The listing builds one solid part. Answer for the finished solid, in the listing's coordinates (mm). Give positions to 0.01 mm unless a question says otherwise; leave off trailing zeros. Order: outer loops, then holes, each group sorted by start corner. A loop starts at its lowest first (then second) coordinate and runs counter-clockwise, first axis right, second up. Notation, with made-up numbers: (65.25, -29) -> (88.25, -29) arc R16 cw to (88.25, -5) -> close; hole circle Ø1 at (39, 28). An arc over 180 degrees is marked (long way). One line per question, with ' | ' between items. Start each with the question number.
```python
from build123d import *

# Parameters (mm, degrees)
SZKIC2_W                   = 5.611911117
SZKIC2_H                   = 18
WYTNIJ_WYCI_GNI_CIE3_DEPTH = 100
SZKIC3_R                   = 4
WYTNIJ_WYCI_GNI_CIE4_DEPTH = 9
WYTNIJ_WYCI_GNI_CIE5_DEPTH = 1
SZKIC5_R                   = 4
WYTNIJ_WYCI_GNI_CIE6_DEPTH = 70


with BuildPart() as part:
    # Szkic1 → Obrót1 (revolve)
    with BuildSketch(Plane.XY):
        with BuildLine():
            Line((0, 0), (-2, 0))
            Line((-2, 0), (-2, 47.515991356))
            Line((-2, 47.515991356), (-4, 47.515991356))
            Line((-4, 47.515991356), (-4, 52.515991356))
            Line((-4, 52.515991356), (-3, 52.515991356))
            Line((-3, 52.515991356), (-3, 72.515991356))
            Line((-3, 72.515991356), (-6.811196546, 79.117177411))
            ThreePointArc((-6.811196546, 79.117177411), (-8.18368509, 88.745303506), (0, 94))
            Line((0, 94), (0, 87.5))
            ThreePointArc((0, 87.5), (-2.5, 85), (0, 82.5))
            Line((0, 82.5), (0, 0))
        make_face()
    revolve(axis=Axis((0, 82.5, 0), (0, -1, 0)))

    # Szkic2 → Wytnij-wyciągnięcie3 (cut)
    with BuildSketch(Plane(origin=(0, 0, 0), x_dir=(1, 0, 0), z_dir=(0, 1, 0))):
        with Locations((-6.805955559, 0)):
            Rectangle(SZKIC2_W, SZKIC2_H)
        with Locations((6.805955559, 0)):
            Rectangle(SZKIC2_W, SZKIC2_H)
    extrude(amount=WYTNIJ_WYCI_GNI_CIE3_DEPTH, mode=Mode.SUBTRACT)

    # Szkic3 → Wytnij-wyciągnięcie4 (cut, through all)
    with BuildSketch(Plane.ZY.offset(4)):
        with Locations((0, 85)):
            Circle(SZKIC3_R)
    extrude(amount=-WYTNIJ_WYCI_GNI_CIE4_DEPTH, mode=Mode.SUBTRACT)

    # Szkic4 → Wytnij-wyciągnięcie5 (cut)
    with BuildSketch(Plane.ZY.offset(4)):
        with BuildLine():
            ThreePointArc((6.270693727, 78.457606273), (-1.54e-07, 94.062257748), (-6.270693505, 78.45760606))
            add(Edge.make_bspline(
                [(-6.270693505, 78.45760606), (-5.860155238, 77.884005031), (-5.439822901, 77.318273551), (-4.56334323, 76.215587996), (-4.106381954, 75.67754923), (-3.363374021, 74.922329572), (-3.10680463, 74.680734677), (-2.565651322, 74.22947798), (-2.278481074, 74.018621845), (-1.674076312, 73.65846472), (-1.356546022, 73.509032989), (-0.676664628, 73.299784881), (-0.328815369, 73.245372297), (0.202925796, 73.249526844), (0.380729476, 73.265518373), (0.727839454, 73.323535586), (0.898553898, 73.365855519), (1.234860958, 73.474497232), (1.400715996, 73.541171917), (1.719331355, 73.691591375), (1.873358854, 73.775663717), (2.32266111, 74.049331959), (2.606912587, 74.261443159), (3.145505929, 74.716004998), (3.399015103, 74.956985507), (4.130320647, 75.70528438), (4.580547786, 76.236525924), (5.447234702, 77.328310614), (5.863652605, 77.888890096), (6.270693727, 78.457606273)],
                knots=[0, 0, 0, 0, 0.125, 0.125, 0.25, 0.25, 0.3125, 0.3125, 0.375, 0.375, 0.4375, 0.4375, 0.5, 0.5, 0.53125, 0.53125, 0.5625, 0.5625, 0.59375, 0.59375, 0.625, 0.625, 0.6875, 0.6875, 0.75, 0.75, 0.875, 0.875, 1, 1, 1, 1], degree=3))
        make_face()
    wytnij_wyci_gni_cie5 = extrude(amount=-WYTNIJ_WYCI_GNI_CIE5_DEPTH, mode=Mode.SUBTRACT)

    # Lustro1: Wytnij-wyciągnięcie5 across plane
    add(wytnij_wyci_gni_cie5.mirror(Plane(origin=(0, 0, 0), x_dir=(0, 0, 1), z_dir=(1, 0, 0))), mode=Mode.SUBTRACT)

    # Szkic5 → Wytnij-wyciągnięcie6 (cut)
    with BuildSketch(Plane(origin=(0, 0, 0), x_dir=(1, 0, 0), z_dir=(0, 1, 0))):
        Circle(SZKIC5_R)
    extrude(amount=WYTNIJ_WYCI_GNI_CIE6_DEPTH, mode=Mode.SUBTRACT)


solid = part.part
```
(1) Determine the mould class of faces 1 (the face through (3, 71, 0)), 2 (the face through (0, 70, 0)), 3 (the face through (-0.042, 81.095, -0.867)) for opening direction Z: pulls with the +Z half, pulls with the -Z half, needs draft (parallel to the pull), parting line crosses it, or undercut.
(2) Given P1, Ø2, axis at x = 0, y = 74.5, coming from the +Z side; P2, Ø3, axis at x = 1, z = -3.5, coming from the +Y side; P3, Ø2, axis at x = -0.5, y = 81.5, coming from the -Z side, each flat-ended and moving along its own axis, determine where each tip first touches the part or whether it passes through.
(3) Consider line 1 (Y direction, x = 0.3, z = 0) (3 decimals); line 2 (X direction, y = 78.5, z = 1); line 3 (Y direction, x = 2.5, z = 1.75). Determine where each line is inside the solid, lowest interval first.
(4) The part is cut by section B-B on y = 85. Determine the outline of the cut face in (x, z).
(5) The part is cut by section C-C on y = 82.5. Determine the outline of the cut face in (x, z), plus the area to 3 significant figures.
(6) The part is cut by section A-A on x = 0. Determine the outline of the cut face in (y, z), plus the area to 3 significant figures.
Result sheet:
1) face 1: parting line crosses it | face 2: needs draft | face 3: undercut
2) P1: stops at z = 4.72 | P2: stops at y = 93.74 | P3: stops at z = -8.64
3) line 1: y = 70 to 81, 89 to 93.995 | line 2: x = -3 to 3 | line 3: y = 72.61 to 81.4, 88.6 to 93.47
4) outline: (-3, -8.49) arc R9 ccw to (3, -8.49) -> (3, -4) -> (-3, -4) -> close; (-3, 4) -> (3, 4) -> (3, 8.49) arc R9 ccw to (-3, 8.49) -> close
5) outline: (-3, -8.11) arc R8.65 ccw to (3, -8.11) -> (3, -3.12) -> (-3, -3.12) -> close; (-3, 3.12) -> (3, 3.12) -> (3, 8.11) arc R8.65 ccw to (-3, 8.11) -> close | area: 64.2 mm^2
6) outline: (70, -3) -> (72.52, -3) -> (79.12, -6.81) arc R9 ccw (long way) to (79.12, 6.81) -> (72.52, 3) -> (70, 3) -> close; hole circle Ø8 at (85, 0) | area: 255 mm^2
